Design review of the part built by this model. Coordinates are the model's own, in mm. Face numbers are marked on the shaded views. Round coordinates to 2 decimals unless told otherwise and drop trailing zeros. Write item = value, one per line.
from build123d import *

# Parameters (mm, degrees)
F0_R     = 15
F0_R_2   = 10
F1_DEPTH = 25
F2_DEPTH = 25
F3_R     = 2
F4_SIZE  = 3


with BuildPart() as f1:
    # F0 (on Front) → F1 (new body)
    with BuildSketch(Plane.XZ):
        with BuildLine():
            ThreePointArc((6.25, -29.341736), (23.318448, -18.874586), (30, 0))
            ThreePointArc((30, 0), (23.318448, 18.874586), (6.25, 29.341736))
            ThreePointArc((6.25, 29.341736), (-30, 0), (6.25, -29.341736))
        make_face()
        Circle(F0_R, mode=Mode.SUBTRACT)
        with BuildLine():
            ThreePointArc((6.25, 29.341736), (23.318448, 18.874586), (30, 0))
            ThreePointArc((30, 0), (23.318448, -18.874586), (6.25, -29.341736))
            Line((6.25, -29.341736), (63.645833, -17.116013))
            ThreePointArc((63.645833, -17.116013), (42.5, 0), (63.645833, 17.116013))
            Line((63.645833, 17.116013), (6.25, 29.341736))
        make_face()
        with BuildLine():
            ThreePointArc((77.5, 0), (73.602428, 11.010175), (63.645833, 17.116013))
            ThreePointArc((63.645833, 17.116013), (42.5, 0), (63.645833, -17.116013))
            ThreePointArc((63.645833, -17.116013), (73.602428, -11.010175), (77.5, 0))
        make_face()
        with Locations((60, 0)):
            Circle(F0_R_2, mode=Mode.SUBTRACT)
    extrude(amount=F1_DEPTH)

    # F0 (on Front) → F2 (join)
    with BuildSketch(Plane.XZ):
        with BuildLine():
            ThreePointArc((6.25, -29.341736), (23.318448, -18.874586), (30, 0))
            ThreePointArc((30, 0), (23.318448, 18.874586), (6.25, 29.341736))
            ThreePointArc((6.25, 29.341736), (-30, 0), (6.25, -29.341736))
        make_face()
        Circle(F0_R, mode=Mode.SUBTRACT)
    extrude(amount=-F2_DEPTH)

    # F3
    f3_edges = [f1.edges().sort_by_distance(p)[0] for p in [
        (-6.25, 25, 29.341736),
        (34.947917, -25, 23.228875),
    ]]
    fillet(f3_edges, radius=F3_R)

    # F4
    f4_edges = [f1.edges().sort_by_distance(p)[0] for p in [
        (-15, 25, 0),
        (50, 0, 0),
    ]]
    chamfer(f4_edges, length=F4_SIZE)


solid = f1.part
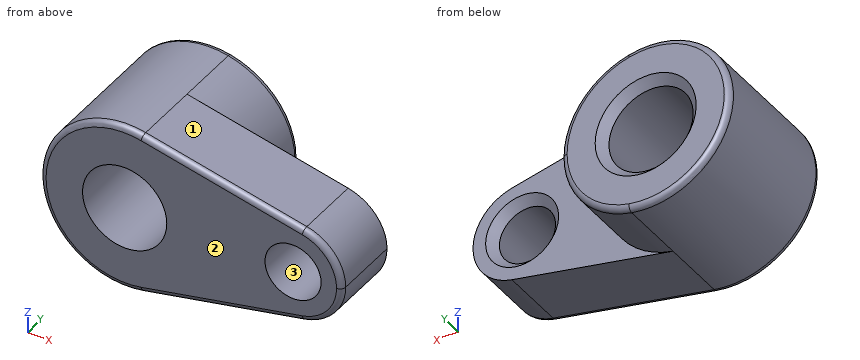
1) We need section A-A on z = -3.5. Give the number of separate pieces and of enclosed holes in the cut face, and give its area (3 significant figures).
Findings:
separate_pieces = 3
enclosed_holes = 0
area = 2,210 mm^2
2) To check wall thickness, follow L1, parallel to X at y = -17.5, z = 9; L2, parallel to X at y = -5, z = 6; L3, parallel to Z at x = 0, y = 5. State the ranges of each line that lie inside material, in increasing order. Write a range as from..to.
Findings:
L1 = -28.62..-12, 12..55.64, 64.36..75.01
L2 = -29.39..-13.75, 13.75..52, 68..76.44
L3 = -30..-15, 15..30
3) Clearance check with flat-ended pins moving along their axes: pin 1 Ø5 at (x, z) = (52, 7.5) entering from +Y; pin 2 Ø23 at (x, z) = (60, 0) entering from +Y; pin 3 Ø5 at (x, y) = (19.5, 18) entering from -Z. State where each tip first meets the part, or that it passes through.
Findings:
pin_1 = 0
pin_2 = -1.5
pin_3 = -24.72
4) The part is to be moulded in two halves that separate along X. For the marked faces 1, 2 and 3, say which applies: released by +X, released by -X, zero draft, split by the parting line, or undercut.
Findings:
face_1 = released by +X
face_2 = zero draft
face_3 = undercut
